Autodesk Inventor part; units mm, degrees
ref_plane "工作平面1" through (0, 0, 0) normal (0, 0, 1) x (1, 0, 0)
ref_plane "YZ Plane" through (0, 0, 0) normal (1, 0, 0) x (0, 1, 0)
ref_plane "XZ Plane" through (0, 0, 0) normal (0, 1, 0) x (-1, 0, 0)
ref_plane "工作平面1" through (0, 0, 0) normal (0, 0, 1) x (1, 0, 0)
sketch "草图1" plane through (0, 0, 0) normal (0, 0, 1) x (1, 0, 0)
  circle A0 centre (0, 0) radius 75
  circle A1 centre (0, 0) radius 100
  circle A2 centre (43.75, 75.7772) radius 5.5
  circle A3 centre (87.5, 0) radius 5.5
  circle A4 centre (-43.75, -75.7772) radius 5.5
  circle A5 centre (-43.75, 75.7772) radius 5.5
  circle A6 centre (-87.5, 0) radius 5.5
  circle A7 centre (43.75, -75.7772) radius 5.5
  point P0 (0, 0)
extrude "拉伸1" add sketch "草图1" along normal blind 0.18
properties part number "垫片4"
The model under review builds one solid part; all positions refer to its coordinate system, in mm. Round coordinates to 2 decimals unless told otherwise and drop trailing zeros. Order: outer loops, then holes, each group sorted by start corner. A loop starts at its lowest first (then second) coordinate and runs counter-clockwise, first axis right, second up. Notation, with made-up numbers: (-28, 12) -> (6, 12) arc R15 cw to (6, 33) -> close; hole circle Ø4 at (75, 29.5). An arc over 180 degrees is marked (long way). Write item = value, one per line. Start each with the question number.
Item 1: Consider section C-C on y = -26.5. Write out the cut boundary in (x, z), plus the area to 3 significant figures.
Item 2: Consider section B-B on x = 0. Write out the cut boundary in (y, z), plus the area to 3 significant figures.
Item 3: Consider section A-A on y = 0. Write out the cut boundary in (x, z), plus the area to 3 significant figures.
Item 4: For line 1 along X through (y, z) = (0.5, 0.1); line 2 along X through (y, z) = (5, 0.1); line 3 along Y through (x, z) = (67.5, 0.05), list the stretches that pass through material, from the lowest coordinate up.
Item 5: Consider section D-D on z = 0.1. Write out the cut boundary in (x, y), plus the area to 3 significant figures.
Conclusion:
q1.outline = (-96.42, 0) -> (-70.16, 0) -> (-70.16, 0.18) -> (-96.42, 0.18) -> close; (70.16, 0) -> (96.42, 0) -> (96.42, 0.18) -> (70.16, 0.18) -> close
q1.area = 9.45 mm2
q2.outline = (-100, 0) -> (-75, 0) -> (-75, 0.18) -> (-100, 0.18) -> close; (75, 0) -> (100, 0) -> (100, 0.18) -> (75, 0.18) -> close
q2.area = 9.00 mm2
q3.outline = (-100, 0) -> (-93, 0) -> (-93, 0.18) -> (-100, 0.18) -> close; (-82, 0) -> (-75, 0) -> (-75, 0.18) -> (-82, 0.18) -> close; (75, 0) -> (82, 0) -> (82, 0.18) -> (75, 0.18) -> close; (93, 0) -> (100, 0) -> (100, 0.18) -> (93, 0.18) -> close
q3.area = 5.04 mm2
q4.line_1 = -100 to -92.98, -82.02 to -75, 75 to 82.02, 92.98 to 100
q4.line_2 = -99.87 to -89.79, -85.21 to -74.83, 74.83 to 85.21, 89.79 to 99.87
q4.line_3 = -73.78 to -32.69, 32.69 to 73.78
q5.outline = circle Ø200 at (0, 0); hole circle Ø11 at (-87.5, 0); hole circle Ø150 at (0, 0); hole circle Ø11 at (-43.75, -75.78); hole circle Ø11 at (-43.75, 75.78); hole circle Ø11 at (43.75, -75.78); hole circle Ø11 at (43.75, 75.78); hole circle Ø11 at (87.5, 0)
q5.area = 13,200 mm2
